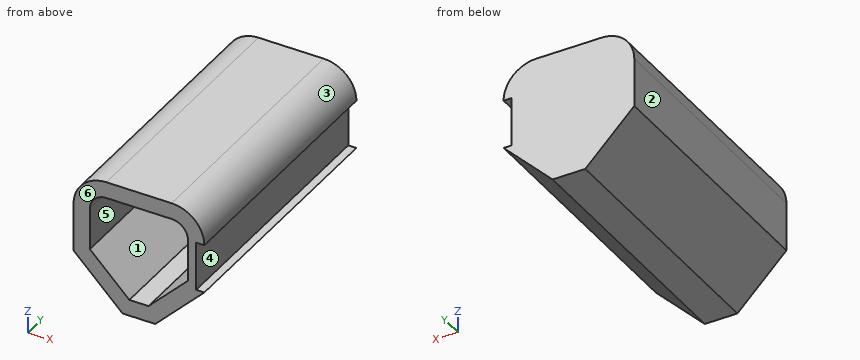
```python
from build123d import *

# Parameters (mm, degrees)
F0_W      = 40
F0_H      = 80
F1_DEPTH  = 40
F2_SIZE   = 15
F3_R      = 10
F4_T      = -5
F1_FACE_W = 80
F1_FACE_H = 15
F5_DEPTH  = 2.5


with BuildPart() as f1:
    # F0 (on Top) → F1 (new body)
    with BuildSketch(Plane.XY):
        Rectangle(F0_W, F0_H)
    extrude(amount=F1_DEPTH)

    # F2
    f2_edges = [f1.edges().sort_by_distance(p)[0] for p in [
        (-20, 0, 0),
        (20, 0, 0),
    ]]
    chamfer(f2_edges, length=F2_SIZE)

    # F3
    f3_edges = [f1.edges().sort_by_distance(p)[0] for p in [
        (-20, 0, 40),
        (20, 0, 40),
    ]]
    fillet(f3_edges, radius=F3_R)

    # F4
    f4_openings = [f1.faces().sort_by_distance(p)[0] for p in [
        (0, -40, 21.961191),
    ]]
    offset(amount=F4_T, openings=f4_openings)

    # F1_face (on face) → F5 (cut)
    with BuildSketch(Plane(origin=(20, 0, 22.5), x_dir=(0, 1, 0), z_dir=(1, 0, 0))):
        Rectangle(F1_FACE_W, F1_FACE_H)
    extrude(amount=-F5_DEPTH, mode=Mode.SUBTRACT)


solid = f1.part
```
Work out the finished part from the listing and answer in its coordinate system (mm). Face numbers are marked on the shaded views. A direction names the side the tool comes from. Give positions to 0.01 mm unless a question says otherwise; leave off trailing zeros. Loops run counter-clockwise (first coordinate to the right, second up) from the corner with the lowest first, then second, coordinate; pieces in that order, holes last. Notation, with made-up numbers: (50, 1.5) -> (80, 1.5) arc R23 ccw to (80, 30.5) -> close; hole circle Ø4 at (64.5, 30). An arc over 180 degrees is marked (long way). Write item = value, one per line. Start each with the question number.
(1) The mould has two halves that part along Z. Classify the marked faces 1, 2, 3 and 4: +Z half, -Z half, draft (parallel to the pull), parting line (faces both ways), or undercut.
(2) Find section D-D on z = 36. Give the vertices of the cut face in (x, y), and give its area (3 significant figures).
(3) Given pin 1 Ø10 at (x, z) = (11.5, 31) entering from -Y; pin 2 Ø12 at (y, z) = (-17.5, 21.5) entering from +X; pin 3 Ø4 at (x, y) = (9.5, 0) entering from -Z; pin 4 Ø2 at (x, y) = (18.5, 8.5) entering from -Z, each flat-ended and moving along its own axis, determine where each tip first touches the part or whether it passes through.
(4) Find the intervals of material crossed by probe 1 along Z at (x, y) = (2.5, -30); probe 2 along X at (y, z) = (-31, 29.5); probe 3 along X at (y, z) = (-25, 7), in increasing order. Write a range as from..to.
(5) Find section C-C on x = 11. Give the vertices of the cut face in (y, z).
(6) Which of the six approach directions +Z, -Z, +X, -X, +Y, -Y give full straight-line access (tool end or side, diameter ignored) to the marked faces 5 and 6?
(7) Find section A-A on z = 19. Give the vertices of the cut face in (x, y).
(8) Find section B-B on y = 5.5. Give the vertices of the cut face in (x, z), and give its area (3 significant figures).
From the geometry:
q1.face_1 = undercut
q1.face_2 = draft
q1.face_3 = +Z half
q1.face_4 = undercut
q2.outline = (-18, -40) -> (18, -40) -> (18, 40) -> (-18, 40) -> close
q2.area = 2,880 mm^2
q3.pin_1 = -40
q3.pin_2 = 17.5
q3.pin_3 = 2.5
q3.pin_4 = 12.5
q4.probe_1 = 0..5, 35..40
q4.probe_2 = -20..-15, 15..17.5
q4.probe_3 = -12..-4.93, 4.93..12
q5.outline = (-40, 6) -> (40, 6) -> (40, 39.95) -> (-40, 39.95) -> (-40, 34.9) -> (35, 34.9) -> (35, 13.07) -> (-40, 13.07) -> close
q6.face_5 = -Y
q6.face_6 = +Z, -Z, +X, -X, -Y
q7.outline = (-20, -40) -> (-15, -40) -> (-15, 35) -> (15, 35) -> (15, -40) -> (17.5, -40) -> (17.5, 40) -> (-20, 40) -> close
q8.outline = (-20, 15) -> (-5, 0) -> (5, 0) -> (20, 15) -> (17.5, 15) -> (17.5, 30) -> (20, 30) arc R10 ccw to (10, 40) -> (-10, 40) arc R10 ccw to (-20, 30) -> close; hole (-15, 17.07) -> (-2.93, 5) -> (2.93, 5) -> (15, 17.07) -> (15, 30) arc R5 ccw to (10, 35) -> (-10, 35) arc R5 ccw to (-15, 30) -> close
q8.area = 551 mm^2
